from build123d import *

# Parameters (mm, degrees)
F0_W     = 50
F0_H     = 50
F0_R     = 1.5
F0_R_2   = 19
F1_DEPTH = 3


with BuildPart() as f1:
    # F0 (on Top) → F1 (new body)
    with BuildSketch(Plane.XY):
        Rectangle(F0_W, F0_H)
        with Locations((-20, -20)):
            Circle(F0_R, mode=Mode.SUBTRACT)
        with Locations((-16, -16)):
            Circle(F0_R, mode=Mode.SUBTRACT)
        with Locations((20, -20)):
            Circle(F0_R, mode=Mode.SUBTRACT)
        with Locations((16, -16)):
            Circle(F0_R, mode=Mode.SUBTRACT)
        with Locations((-16, 16)):
            Circle(F0_R, mode=Mode.SUBTRACT)
        with Locations((-20, 20)):
            Circle(F0_R, mode=Mode.SUBTRACT)
        Circle(F0_R_2, mode=Mode.SUBTRACT)
        with Locations((16, 16)):
            Circle(F0_R, mode=Mode.SUBTRACT)
        with Locations((20, 20)):
            Circle(F0_R, mode=Mode.SUBTRACT)
    extrude(amount=F1_DEPTH)


solid = f1.part
Can you work these out from the model? Positions are in its coordinate system, mm. Give positions to 0.01 mm unless a question says otherwise; leave off trailing zeros. Write each loop counter-clockwise with the first axis right and the second up, starting at its lowest first coordinate (ties: lowest second). Pieces come first, ordered by that corner, then holes. Notation, with made-up numbers: (68.5, -1.75) -> (113.5, -1.75) arc R19 cw to (113.5, 23.25) -> close; hole circle Ø7 at (21, 19.5). An arc over 180 degrees is marked (long way). Answer as a JSON object with one key per item and string values. Group by question number.
Item 1: We'd pull the mould along X, two halves only. Please class faces 1 (the face through (-11, 17, 3)), 2 (the face through (14.5, 16.07, 1.48)), 3 (the face through (25, 0, 1)): +X half, -X half, draft (parallel to the pull), parting line (faces both ways), or undercut.
Item 2: Please list where these lines run through material, in increasing order: line 1 (Y direction, x = 20, z = 2.2); line 2 (Y direction, x = 16, z = 2.3); line 3 (Y direction, x = 20.5, z = 1.1). Write a range as [from, to].
Item 3: Suppose I cut it at A-A (y = 0). Please give me the cut outline in (x, z), plus the area to 3 significant figures.
Item 4: Suppose I cut it at B-B (x = -20). Please give me the cut outline in (y, z), plus the area to 3 significant figures.
Item 5: Suppose I cut it at D-D (y = 16). Please give me the cut outline in (x, z), plus the area to 3 significant figures.
Item 6: I'm going to push a flat-ended pin straight in: P1, Ø5, axis at x = -20, y = 20, coming from the +Z side. Where does the tip first touch, or does it pass through?
Item 7: Suppose I cut it at C-C (z = 1.9). State how many separate pieces and enclosed holes the cut face has, plus the area to 3 significant figures.
Findings:
{
 "1": {"face 1": "draft", "face 2": "undercut", "face 3": "+X half"},
 "2": {"line 1": "y = [-25, -21.5], [-18.5, 18.5], [21.5, 25]", "line 2": "y = [-25, -17.5], [-14.5, -10.25], [10.25, 14.5], [17.5, 25]", "line 3": "y = [-25, -21.41], [-18.59, 18.59], [21.41, 25]"},
 "3": {"outline": "(-25, 0) -> (-19, 0) -> (-19, 3) -> (-25, 3) -> close; (19, 0) -> (25, 0) -> (25, 3) -> (19, 3) -> close", "area": "36.0 mm²"},
 "4": {"outline": "(-25, 0) -> (-21.5, 0) -> (-21.5, 3) -> (-25, 3) -> close; (-18.5, 0) -> (18.5, 0) -> (18.5, 3) -> (-18.5, 3) -> close; (21.5, 0) -> (25, 0) -> (25, 3) -> (21.5, 3) -> close", "area": "132 mm²"},
 "5": {"outline": "(-25, 0) -> (-17.5, 0) -> (-17.5, 3) -> (-25, 3) -> close; (-14.5, 0) -> (-10.25, 0) -> (-10.25, 3) -> (-14.5, 3) -> close; (10.25, 0) -> (14.5, 0) -> (14.5, 3) -> (10.25, 3) -> close; (17.5, 0) -> (25, 0) -> (25, 3) -> (17.5, 3) -> close", "area": "70.5 mm²"},
 "6": {"P1": "stops at z = 3"},
 "7": {"separate pieces": "1", "enclosed holes": "9", "area": "1,310 mm²"}
}
